```python
from build123d import *

# Parameters (mm, degrees)
CROQUIS1_R                               = 220.29375
SALIENTE_EXTRUIR1_DEPTH                  = 0.79375
SALIENTE_EXTRUIR2_START                  = 15.875
CROQUIS2_R                               = 220.29375
CROQUIS2_R_2                             = 219.5
SALIENTE_EXTRUIR2_DEPTH                  = 15.875
SALIENTE_EXTRUIR3_REACH                  = 313.947
SALIENTE_EXTRUIR3_END_RADIUS             = 219.5
SALIENTE_EXTRUIR3_DIRECTION_2_REACH      = 313.947
SALIENTE_EXTRUIR3_DIRECTION_2_END_RADIUS = 219.5
SALIENTE_EXTRUIR4_REACH                  = 496.478
SALIENTE_EXTRUIR4_END_RADIUS             = 220.29375
CROQUIS4_W                               = 27.396001645
CROQUIS4_H                               = 13.46587221


with BuildPart() as part:
    # Croquis1 → Saliente-Extruir1 (new body)
    with BuildSketch(Plane(origin=(0, 0, 0), x_dir=(1, 0, 0), z_dir=(0, 1, 0))):
        with Locations(Location((0, 0, 0), (0, 0, 270))):
            Circle(CROQUIS1_R)
    extrude(amount=SALIENTE_EXTRUIR1_DEPTH)

    # Croquis2 → Saliente-Extruir2 (add)
    with BuildSketch(Plane.XZ.offset(SALIENTE_EXTRUIR2_START)):
        with Locations(Location((0, 0, 0), (0, 0, 270))):
            Circle(CROQUIS2_R)
        with Locations(Location((0, 0, 0), (0, 0, 270))):
            Circle(CROQUIS2_R_2, mode=Mode.SUBTRACT)
    extrude(amount=-SALIENTE_EXTRUIR2_DEPTH)

    # Saliente-Extruir3: up to this cylinder (the profile starts inside it)
    saliente_extruir3_end = Plane(origin=(0, -2.525568, 0), z_dir=(0, 1, 0)) * Cylinder(SALIENTE_EXTRUIR3_END_RADIUS, 1067.894, mode=Mode.PRIVATE)
    # Croquis3 → Saliente-Extruir3 (add, up to the surface)
    with BuildSketch(Plane(origin=(0, 0, 0), x_dir=(0, 0, -1), z_dir=(1, 0, 0)), mode=Mode.PRIVATE) as saliente_extruir3_sk1:
        Polygon((-12.7, 0.79375), (12.7, 0.79375), (12.7, -2.38125), (1.5875, -2.38125), (1.5875, -11.90625), (-1.5875, -11.90625), (-1.5875, -2.38125), (-12.7, -2.38125), align=None)
    saliente_extruir3_tool1 = extrude(saliente_extruir3_sk1.sketch, amount=SALIENTE_EXTRUIR3_REACH, mode=Mode.PRIVATE) & saliente_extruir3_end
    add(saliente_extruir3_tool1.solids().sort_by_distance((0, -2.525568, 0))[0])

    # Saliente-Extruir3 direction 2: up to this cylinder (the profile starts inside it)
    saliente_extruir3_direction_2_end = Plane(origin=(0, -2.525568, 0), z_dir=(0, 1, 0)) * Cylinder(SALIENTE_EXTRUIR3_DIRECTION_2_END_RADIUS, 1067.894, mode=Mode.PRIVATE)
    # Croquis3 → Saliente-Extruir3 direction 2 (add, up to the surface)
    with BuildSketch(Plane(origin=(0, 0, 0), x_dir=(0, 0, -1), z_dir=(1, 0, 0)), mode=Mode.PRIVATE) as saliente_extruir3_direction_2_sk1:
        Polygon((-12.7, 0.79375), (12.7, 0.79375), (12.7, -2.38125), (1.5875, -2.38125), (1.5875, -11.90625), (-1.5875, -11.90625), (-1.5875, -2.38125), (-12.7, -2.38125), align=None)
    saliente_extruir3_direction_2_tool1 = extrude(saliente_extruir3_direction_2_sk1.sketch, amount=-SALIENTE_EXTRUIR3_DIRECTION_2_REACH, mode=Mode.PRIVATE) & saliente_extruir3_direction_2_end
    add(saliente_extruir3_direction_2_tool1.solids().sort_by_distance((0, -2.525568, 0))[0])

    # Saliente-Extruir4: up to this cylinder (the profile starts outside it)
    saliente_extruir4_end = Plane(origin=(0, -6.732936, 0), z_dir=(0, -1, 0)) * Cylinder(SALIENTE_EXTRUIR4_END_RADIUS, 1434.5435, mode=Mode.PRIVATE)
    # Croquis4 → Saliente-Extruir4 (add, up to the surface)
    with BuildSketch(Plane(origin=(-220.262941422, 0, 3.684145126), x_dir=(0.01672378415604664, 0, 0.999860147742424), z_dir=(-0.999860147742424, 0, 0.01672378415604664)), mode=Mode.PRIVATE) as saliente_extruir4_sk1:
        with Locations((1.488935582, -6.732936105)):
            Rectangle(CROQUIS4_W, CROQUIS4_H)
    saliente_extruir4_tool1 = extrude(saliente_extruir4_sk1.sketch, amount=-SALIENTE_EXTRUIR4_REACH, mode=Mode.PRIVATE) - saliente_extruir4_end
    add(saliente_extruir4_tool1.solids().sort_by_distance((-220.238041, -6.732936, 5.172872))[0])
    add(saliente_extruir4_tool1.solids().sort_by_distance((-220.238041, -6.732936, 5.172872))[1])


solid = part.part
```
Build history of the part. All positions in model axes, mm. A direction names the side the tool comes from. Coordinates: 2 decimals unless noted, no trailing zeros. Order: outer loops, then holes, each group sorted by start corner. A loop starts at its lowest first (then second) coordinate and runs counter-clockwise, first axis right, second up.
Item 1: Saw through at C-C on z = -58.5. List the corners of the cut face in (x, y) (3 decimals), then the cut area to 3 significant figures.
Filled in:
outline: (-212.384, -15.875) - (-211.561, -15.875) - (-211.561, 0) - (211.561, 0) - (211.561, -15.875) - (212.384, -15.875) - (212.384, 0.794) - (-212.384, 0.794) - close
area: 363 mm2
Item 2: Drop flat-ended pins along their axis: pin 1 Ø6 at (y, z) = (-10.5, -154) entering from -X; pin 2 Ø7.5 at (x, y) = (112.5, -7) entering from +Z; pin 3 Ø5.5 at (x, z) = (117, -8) entering from -Y. Give the stop position or say it passes through.
Filled in:
pin 1: stops at x = -160.4
pin 2: stops at z = 191.58
pin 3: stops at y = -2.38
Item 3: Drill centre lines: L1, parallel to Z at x = 0, y = -10.5; L2, parallel to Z at x = -5, y = -1; L3, parallel to Y at x = 122.5, z = -149.5. Where is each one in solid material? Low to high.
Filled in:
L1: z = -220.29 to -219.5, -1.59 to 1.59, 219.5 to 220.29
L2: z = -220.24 to -219.44, -12.7 to 12.7, 219.44 to 220.24
L3: y = 0 to 0.79
Item 4: Saw through at D-D on z = 114. List the corners of the cut face in (x, y) (3 decimals), then the cut area to 3 significant figures.
Filled in:
outline: (-188.503, -15.875) - (-187.575, -15.875) - (-187.575, 0) - (187.575, 0) - (187.575, -15.875) - (188.503, -15.875) - (188.503, 0.794) - (-188.503, 0.794) - close
area: 329 mm2
Item 5: Saw through at B-B on x = 63. List the corners of the cut face in (y, z) (1 decimal), then the cut area to 3 significant figures.
Filled in:
outline: (-15.9, -211.1) - (0.8, -211.1) - (0.8, 211.1) - (-15.9, 211.1) - (-15.9, 210.3) - (0, 210.3) - (0, 12.7) - (-2.4, 12.7) - (-2.4, 1.6) - (-11.9, 1.6) - (-11.9, -1.6) - (-2.4, -1.6) - (-2.4, -12.7) - (0, -12.7) - (0, -210.3) - (-15.9, -210.3) - close
area: 452 mm2
Item 6: Tool access for faces 1 (the flat face through (3, 0.794, 3)), 2 (the cylindrical face through (-214.28, -8.05, 47.58)): list every direction of +Z, -Z, +X, -X, +Y, -Y with a clear straight run to the whole face (end or side of a thin tool).
Filled in:
face 1: +Z, -Z, +X, -X, +Y
face 2: -Y
